from build123d import *

# Parameters (mm, degrees)
SKETCH1_W           = 50.8
SKETCH1_H           = 25.4
SKETCH1_R           = 3.2639
BOSS_EXTRUDE1_DEPTH = 3.175
SKETCH2_W           = 50.8
SKETCH2_H           = 3.175
BOSS_EXTRUDE2_DEPTH = 22.225
SKETCH3_R           = 3.2639
CUT_EXTRUDE1_DEPTH  = 22.225
FILLET1_R           = 2.54


with BuildPart() as part:
    # Sketch1 → Boss-Extrude1 (new body)
    with BuildSketch(Plane(origin=(0, 0, 0), x_dir=(1, 0, 0), z_dir=(0, 1, 0))):
        with Locations((25.4, 12.7)):
            Rectangle(SKETCH1_W, SKETCH1_H)
        with Locations((12.7, 12.7)):
            Circle(SKETCH1_R, mode=Mode.SUBTRACT)
        with Locations((38.1, 12.7)):
            Circle(SKETCH1_R, mode=Mode.SUBTRACT)
    extrude(amount=BOSS_EXTRUDE1_DEPTH)

    # Sketch2 → Boss-Extrude2 (add)
    with BuildSketch(Plane(origin=(0, 3.175, 0), x_dir=(1, 0, 0), z_dir=(0, 1, 0))):
        with Locations((25.4, 23.8125)):
            Rectangle(SKETCH2_W, SKETCH2_H)
    extrude(amount=BOSS_EXTRUDE2_DEPTH)

    # Sketch3 → Cut-Extrude1 (cut)
    with BuildSketch(Plane.XY.offset(-22.225)):
        with Locations((38.1, 12.7)):
            Circle(SKETCH3_R)
        with Locations((12.7, 12.7)):
            Circle(SKETCH3_R)
    extrude(amount=-CUT_EXTRUDE1_DEPTH, mode=Mode.SUBTRACT)

    # Fillet1
    fillet1_edges = [part.edges().sort_by_distance(p)[0] for p in [
        (25.4, 3.175, -22.225),
    ]]
    fillet(fillet1_edges, radius=FILLET1_R)


solid = part.part
Design review of the part built by this model. Coordinates are the model's own, in mm. A direction names the side the tool comes from. Coordinates: 2 decimals unless noted, no trailing zeros. Loops run counter-clockwise (first coordinate to the right, second up) from the corner with the lowest first, then second, coordinate; pieces in that order, holes last. Notation, with made-up numbers: M 29,75 L 54,75 A26 ccw 54,104 Z; hole C 89,22 d10. An arc over 180 degrees is marked long. Use one line per item in the form item = value.
(1) For faces 4 (the face through (25, 13, -25.4)), 5 (the face through (25, 15, -22.225)), list the 3-axis set-ups (+Z, -Z, +X, -X, +Y, -Y) from which the entire face can be reached by the end or side of a thin tool; tool diameter is ignored.
Return value:
face_4 = -Z, +X, -X, +Y, -Y
face_5 = +Z, +X, -X, +Y
(2) Consider section C-C (y = 12.7). Write out the cut boundary in (x, z) (3 decimals), and give its area (3 significant figures).
Return value:
outline = M 0,-25.4 L 9.436,-25.4 L 9.436,-22.225 L 0,-22.225 Z; M 15.964,-25.4 L 34.836,-25.4 L 34.836,-22.225 L 15.964,-22.225 Z; M 41.364,-25.4 L 50.8,-25.4 L 50.8,-22.225 L 41.364,-22.225 Z
area = 120 mm2
(3) Draft analysis for pull direction Y (two halves, no side actions). For faces 1 (the face through (41.213, 13.68, -23.79)), 2 (the face through (0, 2, -18)), 3 (the face through (25, 3.175, -10)), state which applies: pulls with the +Y half, pulls with the -Y half, needs draft (parallel to the pull), parting line crosses it, or undercut.
Return value:
face_1 = undercut
face_2 = needs draft
face_3 = pulls with the +Y half
(4) Consider section A-A (x = 38.1). Write out the cut boundary in (y, z) (3 decimals).
Return value:
outline = M 0,-25.4 L 9.436,-25.4 L 9.436,-22.225 L 5.715,-22.225 A2.54 cw 3.175,-19.685 L 3.175,-15.964 L 0,-15.964 Z; M 0,-9.436 L 3.175,-9.436 L 3.175,0 L 0,0 Z; M 15.964,-25.4 L 25.4,-25.4 L 25.4,-22.225 L 15.964,-22.225 Z
(5) Consider section D-D (z = -23.5). Write out the cut boundary in (x, y), and give its area (3 significant figures).
Return value:
outline = M 0,0 L 50.8,0 L 50.8,25.4 L 0,25.4 Z; hole C 12.7,12.7 d6.53; hole C 38.1,12.7 d6.53
area = 1,220 mm2
(6) For line 1 along Z through (x, y) = (38.1, 1.75); line 2 along Z through (x, y) = (41, 6.5) (3 decimals); line 3 along Y through (x, z) = (12.7, -23.9), list the stretches that pass through material, from the lowest coordinate up. Write a range as from..to.
Return value:
line_1 = -25.4..-15.96, -9.44..0
line_2 = -25.4..-22.225
line_3 = 0..9.44, 15.96..25.4
(7) Clearance check with flat-ended pins moving along their axes: P1, Ø4, axis at y = 5.5, z = -18, coming from the +X side; P2, Ø10, axis at x = 30.5, y = 13.5, coming from the +Z side (3 decimals); P3, Ø8, axis at x = 28, z = -16.5, coming from the +Y side. State where each tip first meets the part, or that it passes through.
Return value:
P1 = through
P2 = -22.225
P3 = 3.31
(8) Consider section B-B (z = -12.7). Write out the cut boundary in (x, y) (3 decimals).
Return value:
outline = M 0,0 L 9.436,0 L 9.436,3.175 L 0,3.175 Z; M 15.964,0 L 34.836,0 L 34.836,3.175 L 15.964,3.175 Z; M 41.364,0 L 50.8,0 L 50.8,3.175 L 41.364,3.175 Z
